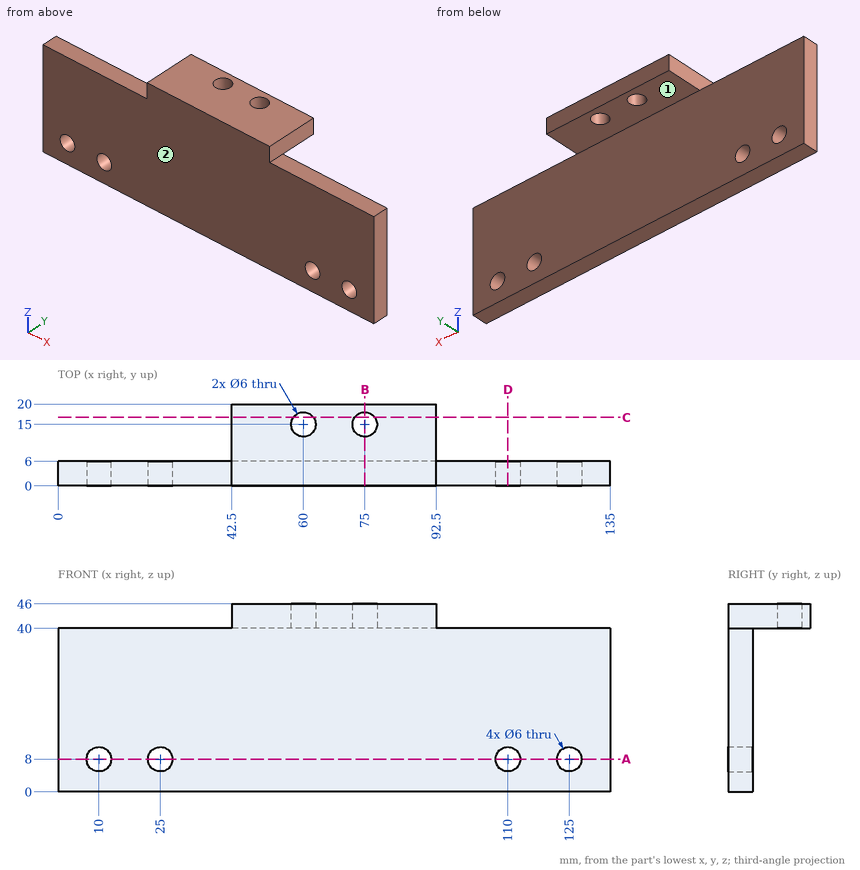
Print and shaded views of the part. All mm, measured from the part's lowest x, y and z. A direction names the side the tool comes from. Coordinates: 2 decimals unless noted, no trailing zeros. Order: outer loops, then holes, each group sorted by start corner. A loop starts at its lowest first (then second) coordinate and runs counter-clockwise, first axis right, second up. Notation, with made-up numbers: M 82,35 L 114,35 A12 ccw 114,49 Z; hole C 57,-39 d9. An arc over 180 degrees is marked long. Answer as CSV lines item,"result".
1) Drill centre lines: L1, parallel to Z at x = 110, y = 2.4; L2, parallel to X at y = 2.5, z = 6; L3, parallel to Y at x = 67, z = 24. Where is each one in solid material? Low to high. Write a range as from..to.
Verdict:
L1,"0..5, 11..40"
L2,"0..7.76, 12.24..22.76, 27.24..107.76, 112.24..122.76, 127.24..135"
L3,"0..6"
2) Cut at D-D (x = 110). List the corners of the cut face in (y, z).
Verdict:
outline,"M 0,0 L 6,0 L 6,5 L 0,5 Z; M 0,11 L 6,11 L 6,40 L 0,40 Z"
3) Cut at C-C (y = 16.75). List the corners of the cut face in (x, z), then the cut area to 3 significant figures.
Verdict:
outline,"M 42.5,40 L 57.56,40 L 57.56,46 L 42.5,46 Z; M 62.44,40 L 72.56,40 L 72.56,46 L 62.44,46 Z; M 77.44,40 L 92.5,40 L 92.5,46 L 77.44,46 Z"
area,"242 mm2"
4) Cut at A-A (z = 8). List the corners of the cut face in (x, y).
Verdict:
outline,"M 0,0 L 7,0 L 7,6 L 0,6 Z; M 13,0 L 22,0 L 22,6 L 13,6 Z; M 28,0 L 107,0 L 107,6 L 28,6 Z; M 113,0 L 122,0 L 122,6 L 113,6 Z; M 128,0 L 135,0 L 135,6 L 128,6 Z"
5) Flat gauge pins, fed straight in: P1, Ø5.5, axis at x = 125, z = 8, coming from the -Y side; P2, Ø1.8, axis at y = 14.5, z = 42.5, coming from the +X side; P3, Ø9.5, axis at x = 110, z = 8, coming from the +Y side; P4, Ø5, axis at y = 11, z = 44, coming from the -X side. Where does each tip first touch, or does it go through?
Verdict:
P1,"through"
P2,"x = 92.5"
P3,"y = 6"
P4,"x = 42.5"
6) 3-axis set-ups, long thin cutter, end or side, ignore diameter. For the marked faces 1 and 2: which of +Z, -Z, +X, -X, +Y, -Y reach the whole face in a straight line?
Verdict:
face 1,"-Z, +X, -X, +Y"
face 2,"+Z, -Z, +X, -X, -Y"
7) Cut at B-B (x = 75). List the corners of the cut face in (y, z), then the cut area to 3 significant figures.
Verdict:
outline,"M 0,0 L 6,0 L 6,40 L 12,40 L 12,46 L 0,46 Z; M 18,40 L 20,40 L 20,46 L 18,46 Z"
area,"324 mm2"
